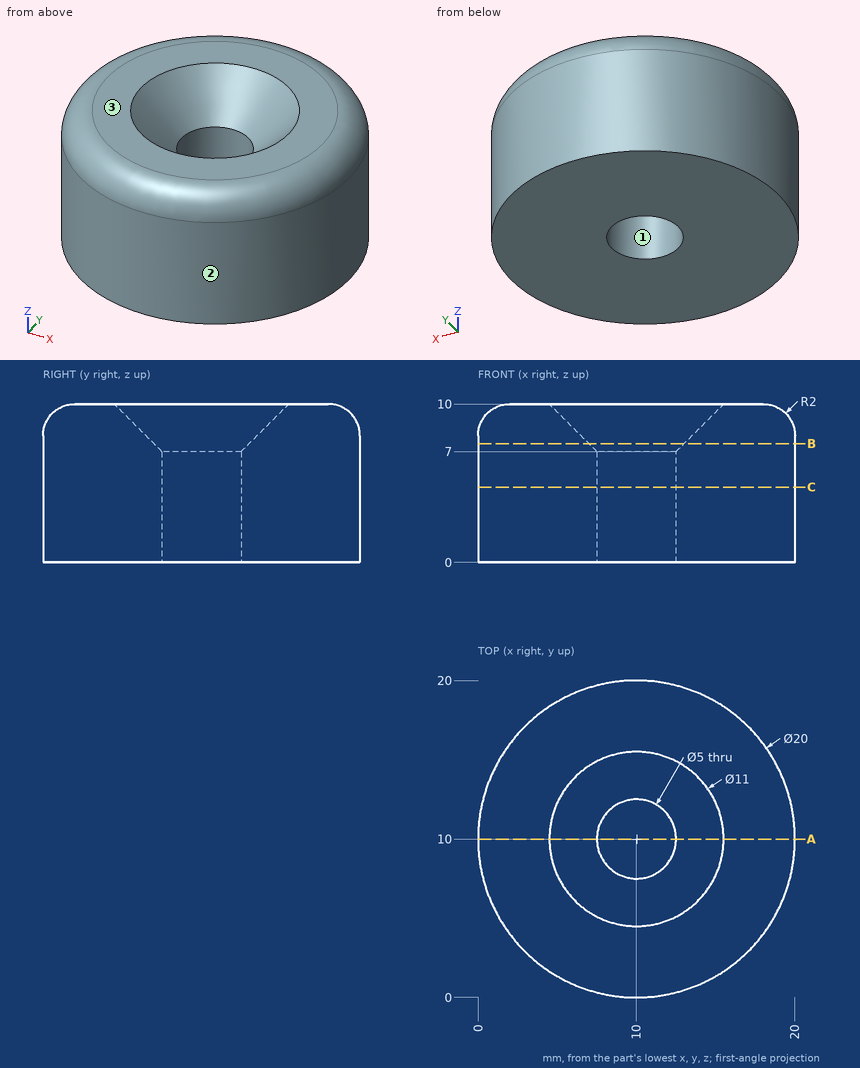
Geometry: see drawing. Coordinates: mm, zero at the bounding-box minimum. Round coordinates to 2 decimals unless told otherwise and drop trailing zeros. Loops run counter-clockwise (first coordinate to the right, second up) from the corner with the lowest first, then second, coordinate; pieces in that order, holes last. Notation, with made-up numbers: (18, -20) - (65, -20) arc R21 ccw to (65, 18) - close; hole circle Ø9 at (-3, -22.75). An arc over 180 degrees is marked (long way). Write item = value, one per line. Start each with the question number.
(1) Pin query (flat end, axial travel): pin 1 (5 mm diameter, centred on y = 17, z = 2, fed in from -X); pin 2 (4 mm diameter, centred on x = 10, y = 10, fed in from +Z); pin 3 (1 mm diameter, centred on x = 5.5, z = 1.5, fed in from +Y); pin 4 (5 mm diameter, centred on y = 4.5, z = 6.5, fed in from -X). Return the tip coordinate at first contact, or that it passes through.
(2) Ray query, line 1 along Y through (x, z) = (10, 3); line 2 along Z through (x, y) = (1.5, 12.25); line 3 along Y through (x, z) = (10, 9.25). Return the intervals inside material, ascending. Write a range as from..to.
(3) Section query A-A, the plane y = 10. Output: boundary loops of the cut face in (x, z), plus the area to 3 significant figures.
(4) Pull-direction query (X, two-part tool) for the marked faces 1, 2 and 3; classes: +X half, -X half, draft (parallel to the pull), parting line (faces both ways), or undercut.
(5) Section query C-C, the plane z = 4.75. Output: boundary loops of the cut face in (x, y).
(6) Section query B-B, the plane z = 7.5. Output: boundary loops of the cut face in (x, y).
Conclusion:
q1.pin_1 = 1.07
q1.pin_2 = through
q1.pin_3 = 19.17
q1.pin_4 = 0.46
q2.line_1 = 0..7.5, 12.5..20
q2.line_2 = 0..9.84
q2.line_3 = 0.44..5.25, 14.75..19.56
q3.outline = (0, 0) - (7.5, 0) - (7.5, 7) - (4.5, 10) - (2, 10) arc R2 ccw to (0, 8) - close; (12.5, 0) - (20, 0) - (20, 8) arc R2 ccw to (18, 10) - (15.5, 10) - (12.5, 7) - close
q3.area = 139 mm2
q4.face_1 = undercut
q4.face_2 = parting line
q4.face_3 = draft
q5.outline = circle Ø20 at (10, 10); hole circle Ø5 at (10, 10)
q6.outline = circle Ø20 at (10, 10); hole circle Ø6 at (10, 10)
